```python
from build123d import *

# Parameters (mm, degrees)
SKETCH7_W          = 7.5
SKETCH7_H          = 9
CUT_EXTRUDE1_DEPTH = 5
SHAFT_HOLE_DEPTH   = 50.734294003


with BuildPart() as part:
    # Sketch2 → Revolve1 (revolve)
    with BuildSketch(Plane(origin=(0, 0, 0), x_dir=(0, 0, -1), z_dir=(1, 0, 0)), mode=Mode.PRIVATE) as revolve1_sk:
        Polygon((0, 0), (0, 32.5), (-8.25, 32.5), (-8.25, 27.5), (-10.75, 27.5), (-10.75, 32.5), (-19, 32.5), (-19, 25.5), (-5, 25.5), (-5, 0), align=None)
    revolve(revolve1_sk.sketch.rotate(Axis((0, 0, 5), (0, 0, -1)), 90), axis=Axis((0, 0, 5), (0, 0, -1)))

    # Sketch7 → Cut-Extrude1 (cut)
    with BuildSketch(Plane(origin=(0, 32.5, 0), x_dir=(1, 0, 0), z_dir=(0, 1, 0))):
        with Locations((0, -9.5)):
            Rectangle(SKETCH7_W, SKETCH7_H)
    cut_extrude1 = extrude(amount=-CUT_EXTRUDE1_DEPTH, mode=Mode.SUBTRACT)

    # Mirror1: Cut-Extrude1 across plane
    add(cut_extrude1.mirror(Plane.ZX), mode=Mode.SUBTRACT)

    # Sketch8 → Shaft Hole (cut, through all)
    with BuildSketch(Plane(origin=(0, 0, 0), x_dir=(-1, 0, 0), z_dir=(0, 0, -1))):
        with BuildLine():
            Line((-1.378404875, 1.65), (1.378404875, 1.65))
            ThreePointArc((1.378404875, 1.65), (0, -2.15), (-1.378404875, 1.65))
        make_face()
    extrude(amount=-SHAFT_HOLE_DEPTH, mode=Mode.SUBTRACT)


solid = part.part
```
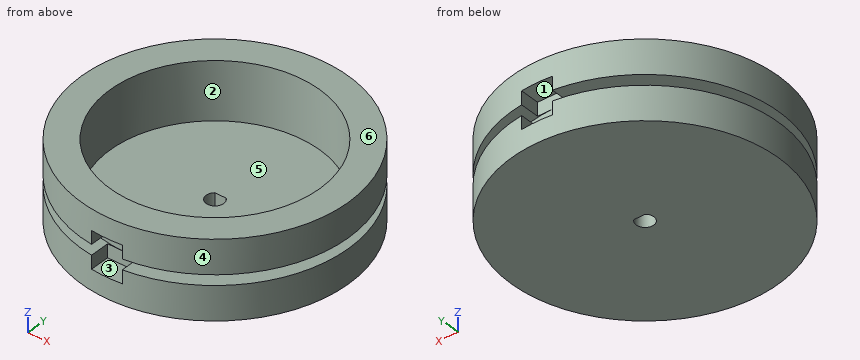
Geometry: final body of the model. Coordinates: model frame, mm. Face numbers are marked on the shaded views. A direction names the side the tool comes from. Round coordinates to 2 decimals unless told otherwise and drop trailing zeros. Loops run counter-clockwise (first coordinate to the right, second up) from the corner with the lowest first, then second, coordinate; pieces in that order, holes last.
Item 1: Mould query, pull axis X, two halves, no side actions, for the marked faces 4, 5 and 6. Classes: released by +X, released by -X, zero draft, split by the parting line, or undercut.
Checked values:
face 4: split by the parting line
face 5: undercut
face 6: zero draft
Item 2: Section B-B, the plane z = 12. Output: boundary loops of the cut face in (x, y).
Checked values:
outline: (-3.75, -32.28) - (-3.75, -27.5) - (3.75, -27.5) - (3.75, -32.28) arc R32.5 ccw to (3.75, 32.28) - (3.75, 27.5) - (-3.75, 27.5) - (-3.75, 32.28) arc R32.5 ccw to start; hole circle Ø51 at (0, 0)
Item 3: Section A-A, the plane y = 0. Output: boundary loops of the cut face in (x, z).
Checked values:
outline: (-32.5, 0) - (-2.15, 0) - (-2.15, 5) - (-25.5, 5) - (-25.5, 19) - (-32.5, 19) - (-32.5, 10.75) - (-27.5, 10.75) - (-27.5, 8.25) - (-32.5, 8.25) - close; (2.15, 0) - (32.5, 0) - (32.5, 8.25) - (27.5, 8.25) - (27.5, 10.75) - (32.5, 10.75) - (32.5, 19) - (25.5, 19) - (25.5, 5) - (2.15, 5) - close
Item 4: Line query: L1, parallel to Z at x = 22, y = 21.5; L2, parallel to Y at x = 0, z = 14.25; L3, parallel to Y at x = 0, z = 9.75. Output: solid intervals per line, ascending.
Checked values:
L1: z = 0 to 8.25, 10.75 to 19
L2: y = -32.5 to -25.5, 25.5 to 32.5
L3: y = -27.5 to -25.5, 25.5 to 27.5
Item 5: Reachability of the marked faces 1, 2 and 3 from +Z, -Z, +X, -X, +Y, -Y: full face, straight path, thin tool, end or side. Return the list, or none.
Checked values:
face 1: +Y
face 2: +Z
face 3: -Y
Item 6: Section C-C, the plane x = -8. Output: boundary loops of the cut face in (y, z).
Checked values:
outline: (-31.5, 0) - (31.5, 0) - (31.5, 8.25) - (26.31, 8.25) - (26.31, 10.75) - (31.5, 10.75) - (31.5, 19) - (24.21, 19) - (24.21, 5) - (-24.21, 5) - (-24.21, 19) - (-31.5, 19) - (-31.5, 10.75) - (-26.31, 10.75) - (-26.31, 8.25) - (-31.5, 8.25) - close
Item 7: Contact query for flat-ended pins moving along their axis: P1, Ø2, axis at x = 7, z = 12, coming from the -Y side; P2, Ø1.6, axis at y = 30, z = 13, coming from the +X side; P3, Ø5, axis at x = -25, z = 9.5, coming from the +Y side. Output: stop coordinate, or through.
Checked values:
P1: stops at y = -31.94
P2: stops at x = 14.27
P3: stops at y = 23.13
Item 8: Section D-D, the plane y = -16. Output: boundary loops of the cut face in (x, z).
Checked values:
outline: (-28.29, 0) - (28.29, 0) - (28.29, 8.25) - (22.37, 8.25) - (22.37, 10.75) - (28.29, 10.75) - (28.29, 19) - (19.86, 19) - (19.86, 5) - (-19.86, 5) - (-19.86, 19) - (-28.29, 19) - (-28.29, 10.75) - (-22.37, 10.75) - (-22.37, 8.25) - (-28.29, 8.25) - close
